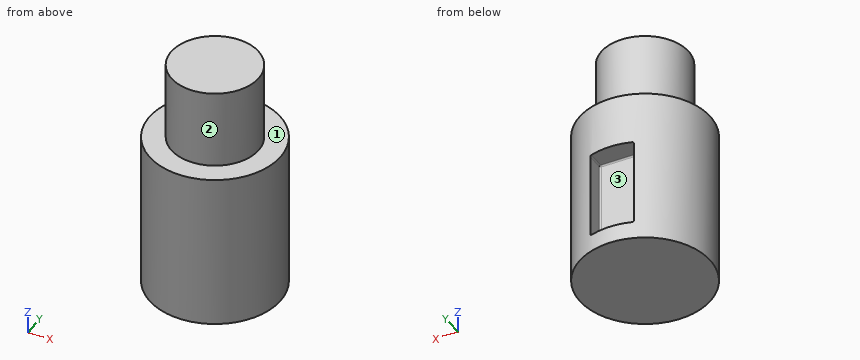
Autodesk Inventor part; units mm, degrees
ref_plane "YZ Plane" through (0, 0, 0) normal (1, 0, 0) x (0, 1, 0)
ref_plane "XY Plane" through (0, 0, 0) normal (0, 0, 1) x (1, 0, 0)
sketch "草圖2" plane through (0, 0, 0) normal (0, 0, 1) x (1, 0, 0)
  circle A0 centre (0, 0) radius 7.5
  dimension "d3" = 15
extrude "擠出2" add sketch "草圖2" along normal blind 18
sketch "草圖3" plane through (0, 0, 18) normal (0, 0, 1) x (1, 0, 0)
  circle A0 centre (0, 0) radius 5
  dimension "d6" = 10
extrude "擠出3" add sketch "草圖3" along normal blind 9
ref_plane "工作平面2" through (0, 7.5, 0) normal (0, 1, 0) x (-1, 0, 0)
sketch "草圖6" plane through (0, 7.5, 0) normal (0, 1, 0) x (-1, 0, 0)
  line L0 (-2.5, 12) -> (2.5, 12)
  line L1 (2.5, 12) -> (2.5, 2)
  line L2 (2.5, 2) -> (-2.5, 2)
  line L3 (-2.5, 2) -> (-2.5, 12)
  line L4 (-2.5, 12) -> (2.5, 2) construction
  line L5 (2.5, 12) -> (-2.5, 2) construction
  line L6 (-7.5, 0) -> (7.5, 0)
  point P0 (0, 0)
  point P1 (0, 7)
  dimension "d24" = 5
  dimension "d25" = 10
  dimension "d26" = 2
  dimension "d27" = 5
extrude "擠出6" cut sketch "草圖6" against normal blind 2.5
fillet "圓角3" radius 0.16 8 edges at (0, 5, 12) (2.5, 6.0355, 12) (2.5, 5, 7) (-2.5, 6.0355, 12) (-2.5, 5, 7) (-2.5, 6.0355, 2) (0, 5, 2) (2.5, 6.0355, 2)
properties part number "軸1"
Verification items for the finished model (mm, model axes). Face numbers are marked on the shaded views. Coordinates: 2 decimals unless noted, no trailing zeros. Write each loop counter-clockwise with the first axis right and the second up, starting at its lowest first coordinate (ties: lowest second). Pieces come first, ordered by that corner, then holes. Notation, with made-up numbers: M 23,-7 L 50,-7 A3 ccw 50,-3 Z; hole C -15.75,84 d8. An arc over 180 degrees is marked long. Answer as a JSON object with one key per item and string values. Group by question number.
(1) Cross-section at C-C, the plane z = 2.5. Record the cut outline in (x, y), and give its area (3 significant figures).
(2) Gauge pin test, flat ends, axial feed: pin 1 (6 mm diameter, centred on y = -4, z = 14.5, fed in from +X); pin 2 (1.5 mm diameter, centred on y = 6.5, z = 9, fed in from -X); pin 3 (3 mm diameter, centred on y = -5, z = 3.5, fed in from +X). Record the tip position at first contact, or that the pin passes through.
(3) Cross-section at B-B, the plane y = 0. Record the cut outline in (x, z).
(4) Material ranges on line 1 (Z direction, x = -1.75, y = 5.5); line 2 (Z direction, x = -5, y = 2.5); line 3 (X direction, y = 5.5, z = 10), recorded low to high.
(5) Release check for a two-part mould opening along Z. For the marked faces 1, 2 and 3 record: +Z half, -Z half, draft (parallel to the pull), parting line (faces both ways), or undercut.
(6) Cross-section at A-A, the plane x = 0. Record the cut outline in (y, z), and give its area (3 significant figures).
(7) Cross-section at D-D, the plane z = 14. Record the cut outline in (x, y).
Reply:
{
 "1": {"outline": "M -2.5,5.16 L -2.5,7.07 A7.5 ccw long 2.5,7.07 L 2.5,5.16 A0.16 cw 2.34,5 L -2.34,5 A0.16 cw Z", "area": "165 mm²"},
 "2": {"pin 1": "x = 7.43", "pin 2": "x = -4.82", "pin 3": "x = 6.63"},
 "3": {"outline": "M -7.5,0 L 7.5,0 L 7.5,18 L 5,18 L 5,27 L -5,27 L -5,18 L -7.5,18 Z"},
 "4": {"line 1": "0 to 2, 12 to 18", "line 2": "0 to 18", "line 3": "-5.1 to -2.5, 2.5 to 5.1"},
 "5": {"face 1": "+Z half", "face 2": "draft", "face 3": "undercut"},
 "6": {"outline": "M -7.5,0 L 7.5,0 L 7.5,2 L 5.16,2 A0.16 cw 5,2.16 L 5,11.84 A0.16 cw 5.16,12 L 7.5,12 L 7.5,18 L 5,18 L 5,27 L -5,27 L -5,18 L -7.5,18 Z", "area": "335 mm²"},
 "7": {"outline": "C 0,0 d15"}
}
